Read the model definition and answer for the solid it produces. Units are mm, in the model's axes. A direction names the side the tool comes from. Coordinates: 2 decimals unless noted, no trailing zeros. Loops run counter-clockwise (first coordinate to the right, second up) from the corner with the lowest first, then second, coordinate; pieces in that order, holes last. Notation, with made-up numbers: M 39,58 L 80,58 A30 ccw 80,86 Z; hole C -19.5,37.5 d7. An arc over 180 degrees is marked long. One line per item, written item: value. Start each with the question number.
```python
from build123d import *

# Parameters (mm, degrees)
DODANIE_WYCI_GNI_CIE1_DEPTH = 36
SZKIC2_R                    = 20
WYTNIJ_WYCI_GNI_CIE1_DEPTH  = 36
SFAZOWANIE1_SIZE            = 10
SZKIC3_R                    = 4
WYTNIJ_WYCI_GNI_CIE2_DEPTH  = 18


with BuildPart() as part:
    # Szkic1 → Dodanie-wyciągnięcie1 (new body)
    with BuildSketch(Plane.XY):
        Polygon((0, 0), (86, 0), (86, 15), (71, 15), (71, 75), (15, 75), (15, 15), (0, 15), align=None)
    extrude(amount=DODANIE_WYCI_GNI_CIE1_DEPTH)

    # Szkic2 → Wytnij-wyciągnięcie1 (cut)
    with BuildSketch(Plane.XY.offset(36)):
        with Locations((43, 47.5)):
            Circle(SZKIC2_R)
    extrude(amount=-WYTNIJ_WYCI_GNI_CIE1_DEPTH, mode=Mode.SUBTRACT)

    # Sfazowanie1
    sfazowanie1_edges = [part.edges().sort_by_distance(p)[0] for p in [
        (15, 75, 18),
        (71, 75, 18),
    ]]
    chamfer(sfazowanie1_edges, length=SFAZOWANIE1_SIZE)

    # Szkic3 → Wytnij-wyciągnięcie2 (cut)
    with BuildSketch(Plane(origin=(0, 15, 0), x_dir=(1, 0, 0), z_dir=(0, 1, 0))):
        with Locations((79, -8)):
            Circle(SZKIC3_R)
        with Locations((7, -8)):
            Circle(SZKIC3_R)
        with Locations((79, -28)):
            Circle(SZKIC3_R)
        with Locations((7, -28)):
            Circle(SZKIC3_R)
    extrude(amount=-WYTNIJ_WYCI_GNI_CIE2_DEPTH, mode=Mode.SUBTRACT)


solid = part.part
```
1) Section B-B (z = 28) is taken. Determine the outline of the cut face in (x, y), then the cut area to 3 significant figures.
2) For a pull along Z with two mould halves and no side action, classify faces 1 (the face through (66, 70, 18)), 2 (the face through (42, 21, 0)), 3 (the face through (6.479, 7.605, 24.034)), 4 (the face through (75, 8, 8)) as released by +Z, released by -Z, zero draft, split by the parting line, or undercut.
3) Consider line 1 along X through (y, z) = (6, 28); line 2 along Z through (x, y) = (79, 12); line 3 along Y through (x, z) = (43, 15). Determine where each line is inside the solid, lowest interval first.
4) A tool of negligible diameter and unlimited length cuts with its end or side. For faces 5 (the face through (15, 40, 18)), 6 (the face through (42, 21, 36)), 7 (the face through (71, 40, 18)), from which of +Z, -Z, +X, -X, +Y, -Y can it reach the whole face along a straight path? Write none if from no direction.
5) Section A-A (x = 43) is taken. Determine the outline of the cut face in (y, z).
6) Section D-D (z = 16.5) is taken. Determine the outline of the cut face in (x, y).
7) Flat-ended cylindrical pins translate along their axes: pin 1 (7 mm diameter, centred on x = 79, z = 8, fed in from -Y); pin 2 (8 mm diameter, centred on y = 41.5, z = 14.5, fed in from -X); pin 3 (3 mm diameter, centred on x = 17.5, z = 5.5, fed in from +Y); pin 4 (5 mm diameter, centred on y = 60.5, z = 6.5, fed in from +X). Find the tip coordinate at first contact, or state that the pin passes through.
8) Section C-C (y = 47.5) is taken. Determine the outline of the cut face in (x, z).
Results found:
1. outline: M 0,0 L 3,0 L 3,15 L 0,15 Z; M 11,0 L 75,0 L 75,15 L 71,15 L 71,65 L 61,75 L 25,75 L 15,65 L 15,15 L 11,15 Z; M 83,0 L 86,0 L 86,15 L 83,15 Z; hole C 43,47.5 d40
1. area: 3,050 mm²
2. face 1: zero draft
2. face 2: released by -Z
2. face 3: undercut
2. face 4: undercut
3. line 1: x = 0 to 3, 11 to 75, 83 to 86
3. line 2: z = 0 to 4, 12 to 24, 32 to 36
3. line 3: y = 0 to 27.5, 67.5 to 75
4. face 5: +Z, -Z, -X, +Y
4. face 6: +Z, +X, -X, +Y, -Y
4. face 7: +Z, -Z, +X, +Y
5. outline: M 0,0 L 27.5,0 L 27.5,36 L 0,36 Z; M 67.5,0 L 75,0 L 75,36 L 67.5,36 Z
6. outline: M 0,0 L 86,0 L 86,15 L 71,15 L 71,65 L 61,75 L 25,75 L 15,65 L 15,15 L 0,15 Z; hole C 43,47.5 d40
7. pin 1: passes through
7. pin 2: stops at x = 15
7. pin 3: stops at y = 69
7. pin 4: stops at x = 71
8. outline: M 15,0 L 23,0 L 23,36 L 15,36 Z; M 63,0 L 71,0 L 71,36 L 63,36 Z
